The model under review builds one solid part; all positions refer to its coordinate system, in mm. A direction names the side the tool comes from. Coordinates: 2 decimals unless noted, no trailing zeros. Write each loop counter-clockwise with the first axis right and the second up, starting at its lowest first coordinate (ties: lowest second). Pieces come first, ordered by that corner, then holes. Notation, with made-up numbers: (-21, 52) - (19, 52) arc R31 cw to (19, 81) - close; hole circle Ø9 at (-18, -13.5). An arc over 180 degrees is marked (long way). Put each result on its own line as item: value.
from build123d import *

# Parameters (mm, degrees)
BLOCOBASE_DEPTH           = 5
SKFIXACAO_R               = 1.7
SKFIXACAO_R_2             = 1.55
FIXACAO_DEPTH             = 5.15
RESSALTOFIXACAO_DEPTH     = 0.15
BOTAO_DEPTH               = 2.15
SKETCH5_W                 = 6.3
SKETCH5_H                 = 1
BASECONECTORNONC_DEPTH    = 10.5
SKDESENHOCONECTORNONC_R   = 0.75
DESENHOCONECTORNONC_DEPTH = 20.5
BASECONECTORCOM_DEPTH     = 3.15
SKDESENHOCONECTORCOM_R    = 0.75
DESENHOCONECTORCOM_DEPTH  = 1
BASECONTATO_DEPTH         = 3.15
SKAPOIOROLO_R             = 0.7
APOIOROLO_DEPTH           = 1
SKROLO_R                  = 2.5
ROLO_DEPTH                = 4.3


with BuildPart() as part:
    # skBlocoBase → BlocoBase (new body, symmetric)
    with BuildSketch(Plane(origin=(0, 0, 0), x_dir=(0, 0, -1), z_dir=(1, 0, 0))):
        with BuildLine():
            Line((-10.7, 7.95), (10.7, 7.95))
            ThreePointArc((10.7, 7.95), (12.9627417, 7.0127417), (13.9, 4.75))
            Line((13.9, 4.75), (13.9, -4.75))
            ThreePointArc((13.9, -4.75), (12.9627417, -7.0127417), (10.7, -7.95))
            Line((10.7, -7.95), (-10.7, -7.95))
            ThreePointArc((-10.7, -7.95), (-12.9627417, -7.0127417), (-13.9, -4.75))
            Line((-13.9, -4.75), (-13.9, 4.75))
            ThreePointArc((-13.9, 4.75), (-12.9627417, 7.0127417), (-10.7, 7.95))
        make_face()
    extrude(amount=BLOCOBASE_DEPTH, both=True)

    # skFixacao → Fixacao (cut, symmetric)
    with BuildSketch(Plane(origin=(0, 0, 0), x_dir=(0, 0, -1), z_dir=(1, 0, 0))):
        with Locations((-11.125, -5.1)):
            Circle(SKFIXACAO_R)
        with Locations((11.125, 5.1)):
            Circle(SKFIXACAO_R_2)
    extrude(amount=FIXACAO_DEPTH, both=True, mode=Mode.SUBTRACT)

    # skRessaltoFixacao → RessaltoFixacao (add)
    with BuildSketch(Plane(origin=(5, 0, 0), x_dir=(0, 0, -1), z_dir=(1, 0, 0))):
        with BuildLine():
            ThreePointArc((-8.475, -5.525), (-9.353679656, -3.403679656), (-11.475, -2.525))
            Line((-11.475, -2.525), (-13.7, -2.525))
            Line((-13.7, -2.525), (-13.7, -4.75))
            ThreePointArc((-13.7, -4.75), (-12.821320344, -6.871320344), (-10.7, -7.75))
            Line((-10.7, -7.75), (-8.475, -7.75))
            Line((-8.475, -7.75), (-8.475, -5.525))
        make_face()
        with BuildLine():
            ThreePointArc((-9.789845005, -6.152312282), (-10.474438165, -6.670595205), (-11.325, -6.788194302))
            ThreePointArc((-11.325, -6.788194302), (-11.775561835, -3.529404795), (-9.789845005, -6.152312282))
        make_face(mode=Mode.SUBTRACT)
        with BuildLine():
            ThreePointArc((13.775, 4.675), (12.896320344, 6.796320344), (10.775, 7.675))
            Line((10.775, 7.675), (8.55, 7.675))
            Line((8.55, 7.675), (8.55, 5.45))
            ThreePointArc((8.55, 5.45), (9.428679656, 3.328679656), (11.55, 2.45))
            Line((11.55, 2.45), (13.775, 2.45))
            Line((13.775, 2.45), (13.775, 4.675))
        make_face()
        with BuildLine():
            ThreePointArc((12.353274612, 4.1545681), (11.71815932, 3.667986725), (10.925, 3.562957385))
            ThreePointArc((10.925, 3.562957385), (10.53184068, 6.532013275), (12.353274612, 4.1545681))
        make_face(mode=Mode.SUBTRACT)
    ressaltofixacao = extrude(amount=RESSALTOFIXACAO_DEPTH)

    # MirrorRessaltoFixacao: RessaltoFixacao across plane
    add(ressaltofixacao.mirror(Plane(origin=(0, 0, 0), x_dir=(0, 0, 1), z_dir=(1, 0, 0))))

    # skBotao → Botao (add, symmetric)
    with BuildSketch(Plane(origin=(0, 0, 0), x_dir=(0, 0, -1), z_dir=(1, 0, 0))):
        with BuildLine():
            Line((-10.475, 7.95), (-10.475, 8.6))
            ThreePointArc((-10.475, 8.6), (-9.075, 9.6), (-7.675, 8.6))
            Line((-7.675, 8.6), (-7.675, 7.95))
            Line((-7.675, 7.95), (-10.475, 7.95))
        make_face()
    extrude(amount=BOTAO_DEPTH, both=True)

    # Sketch5 → BaseConectorNONC (add)
    with BuildSketch(Plane(origin=(0, 0, -13.9), x_dir=(-1, 0, 0), z_dir=(0, 0, -1))):
        with Locations((0, -3.975)):
            Rectangle(SKETCH5_W, SKETCH5_H)
        with Locations((0, 3.975)):
            Rectangle(SKETCH5_W, SKETCH5_H)
    extrude(amount=BASECONECTORNONC_DEPTH)

    # skDesenhoConectorNONC → DesenhoConectorNONC (cut)
    with BuildSketch(Plane.XZ.offset(4.475)):
        Polygon((2.65, -22.767142952), (1.616967042, -24.4), (3.15, -24.4), (3.15, -18.161236833), (2.65, -18.161236833), align=None)
        Polygon((-3.15, -24.4), (-1.616967042, -24.4), (-2.65, -22.767142952), (-2.65, -18.161236833), (-3.15, -18.161236833), align=None)
        with Locations((0, -22.767142952)):
            Circle(SKDESENHOCONECTORNONC_R)
    extrude(amount=-DESENHOCONECTORNONC_DEPTH, mode=Mode.SUBTRACT)

    # skBaseConectorCOM → BaseConectorCOM (add, symmetric)
    with BuildSketch(Plane(origin=(0, 0, 0), x_dir=(0, 0, -1), z_dir=(1, 0, 0))):
        with BuildLine():
            Line((9.725, -11.25), (0.225, -11.25))
            ThreePointArc((0.225, -11.25), (-0.482106781, -10.957106781), (-0.775, -10.25))
            Line((-0.775, -10.25), (-0.775, -7.95))
            Line((-0.775, -7.95), (0.225, -7.95))
            Line((0.225, -7.95), (0.225, -9.25))
            ThreePointArc((0.225, -9.25), (0.517893219, -9.957106781), (1.225, -10.25))
            Line((1.225, -10.25), (9.725, -10.25))
            Line((9.725, -10.25), (9.725, -11.25))
        make_face()
    extrude(amount=BASECONECTORCOM_DEPTH, both=True)

    # skDesenhoConectorCOM → DesenhoConectorCOM (cut)
    with BuildSketch(Plane.XZ.offset(11.25)):
        Polygon((2.65, -8.092142952), (1.616967042, -9.725), (3.15, -9.725), (3.15, -3.486236833), (2.65, -3.486236833), align=None)
        Polygon((-3.15, -9.725), (-1.616967042, -9.725), (-2.65, -8.092142952), (-2.65, -3.486236833), (-3.15, -3.486236833), align=None)
        with Locations((0, -8.092142952)):
            Circle(SKDESENHOCONECTORCOM_R)
    extrude(amount=-DESENHOCONECTORCOM_DEPTH, mode=Mode.SUBTRACT)

    # skBaseContato → BaseContato (add, symmetric)
    with BuildSketch(Plane(origin=(0, 0, 0), x_dir=(0, 0, -1), z_dir=(1, 0, 0))):
        with BuildLine():
            Line((2.63302332, 7.95), (2.63302332, 8.486635004))
            ThreePointArc((2.63302332, 8.486635004), (2.497665983, 8.828739854), (2.164880406, 8.985619098))
            Line((2.164880406, 8.985619098), (-24.4, 10.681624431))
            Line((-24.4, 10.681624431), (-24.336285828, 11.679592619))
            Line((-24.336285828, 11.679592619), (3.545575005, 9.899506131))
            ThreePointArc((3.545575005, 9.899506131), (3.878360582, 9.742626887), (4.013717919, 9.400522037))
            Line((4.013717919, 9.400522037), (4.013717919, 7.95))
            Line((4.013717919, 7.95), (2.63302332, 7.95))
        make_face()
    extrude(amount=BASECONTATO_DEPTH, both=True)

    # skApoioRolo → ApoioRolo (add)
    with BuildSketch(Plane(origin=(3.15, 0, 0), x_dir=(0, 0, -1), z_dir=(1, 0, 0))):
        with BuildLine():
            ThreePointArc((-21.354211514, 14.486814776), (-22.754211514, 15.886814776), (-24.154211514, 14.486814776))
            Line((-24.154211514, 14.486814776), (-24.336285828, 11.679592619))
            Line((-24.336285828, 11.679592619), (-22.939130364, 11.590392778))
            Line((-22.939130364, 11.590392778), (-21.541974901, 11.501192936))
            Line((-21.541974901, 11.501192936), (-21.365242034, 14.3114187))
            Line((-21.365242034, 14.3114187), (-21.354211514, 14.486814776))
        make_face()
        with Locations((-22.754211514, 14.486814776)):
            Circle(SKAPOIOROLO_R, mode=Mode.SUBTRACT)
    apoiorolo = extrude(amount=-APOIOROLO_DEPTH)

    # MirrorApoioRolo: ApoioRolo across plane
    add(apoiorolo.mirror(Plane(origin=(0, 0, 0), x_dir=(0, 0, 1), z_dir=(1, 0, 0))))

    # skRolo → Rolo (add)
    with BuildSketch(Plane.ZY.offset(-2.15)):
        with Locations((22.754211514, 14.486814776)):
            Circle(SKROLO_R)
    extrude(amount=ROLO_DEPTH)


solid = part.part
1. To check wall thickness, follow probe 1 along Z at (x, y) = (0, -4); probe 2 along Z at (x, y) = (0, 3.7); probe 3 along Y at (x, z) = (2, 11). State the ranges of each line that lie inside material, in increasing order.
Determined:
probe 1: z = -24.4 to -23.52, -22.02 to 9.83, 12.42 to 13.9
probe 2: z = -24.4 to -23.52, -22.02 to -11.79, -10.46 to 13.9
probe 3: y = -7.94 to -6.8, -3.4 to 7.94, 9.83 to 10.83
2. Consider section D-D on z = 2.5. State the section outline as (x, y) points.
Determined:
outline: (-5, -7.95) - (5, -7.95) - (5, 7.95) - (-5, 7.95) - close; (-3.15, 9.28) - (3.15, 9.28) - (3.15, 10.29) - (-3.15, 10.29) - close
3. Consider section A-A on z = -5.5. State the section outline as (x, y) points, plus the area to 3 significant figures.
Determined:
outline: (-5, -7.95) - (5, -7.95) - (5, 7.95) - (-5, 7.95) - close; (-2.65, -11.25) - (2.65, -11.25) - (2.65, -10.25) - (-2.65, -10.25) - close
area: 164 mm^2
4. Consider section B-B on x = 0. Give the number of separate pieces and of enclosed holes in the cut face, plus the area to 3 significant figures.
Determined:
separate pieces: 5
enclosed holes: 2
area: 499 mm^2
5. The part is to be moulded in two halves that separate along Z. For faces 1 (the cylindrical face through (-2.657, 14.219, 22.108)), 2 (the flat face through (0, -9, 0.775)), 3 (the flat face through (2.15, 16.2, 22.7)), 4 (the flat face through (-2.15, 14, 23)), say which applies: +Z half, -Z half, draft (parallel to the pull), parting line (faces both ways), or undercut.
Determined:
face 1: undercut
face 2: +Z half
face 3: draft
face 4: undercut
6. Consider section C-C on y = 1.75. State the section outline as (x, z) points, plus the area to 3 significant figures.
Determined:
outline: (-5, -13.9) - (5, -13.9) - (5, 13.9) - (-5, 13.9) - close
area: 278 mm^2
7. Machinability: for faces 5 (the cylindrical face through (-0.163, -10.757, -8.824)), 6 (the cylindrical face through (0.04, -9.95, -0.51)), 7 (the cylindrical face through (-2.657, 15.886, 22.723)), 8 (the flat face through (-2.15, 11.8, 22.9)), 9 (the flat face through (2.65, -4, -20)), which of the approach directions +Z, -Z, +X, -X, +Y, -Y give a long, thin tool a straight path to every point of the face, cutting with its end or side? Answer none if there is none.
Determined:
face 5: -Y
face 6: -Z, +X, -X
face 7: -X, +Y
face 8: none
face 9: -Z, +X, +Y, -Y
8. For pin 1 Ø0.7 at (x, y) = (-0.5, 8.5) entering from +Z (3 decimals); pin 2 Ø1 at (x, y) = (-3.5, 3.5) entering from -Z; pin 3 Ø0.8 at (y, z) = (-4, -20) entering from +X; pin 4 Ø2.5 at (y, z) = (5.1, -11.125) entering from +X, all flat-tipped, find the tip position at first contact; note any pin that passes through.
Determined:
pin 1: stops at z = 10.475
pin 2: stops at z = -18.16
pin 3: stops at x = 2.65
pin 4: passes through
